```python
from build123d import *

# Parameters (mm, degrees)
SALIENTE_EXTRUIR1_DEPTH = 14
CROQUIS7_W              = 84
CROQUIS7_H              = 14.5
SALIENTE_EXTRUIR6_DEPTH = 3
SALIENTE_EXTRUIR7_DEPTH = 5
REDONDEO1_R             = 2


with BuildPart() as part:
    # Croquis1 → Saliente-Extruir1 (new body)
    with BuildSketch(Plane.XY):
        Polygon((-38.5, 7.25), (-42, 7.25), (-42, -7.25), (42, -7.25), (42, 7.25), (38.5, 7.25), (38.5, -2.25), (-38.5, -2.25), align=None)
    extrude(amount=SALIENTE_EXTRUIR1_DEPTH)

    # Croquis7 → Saliente-Extruir6 (add)
    with BuildSketch(Plane.XY.offset(14)):
        Rectangle(CROQUIS7_W, CROQUIS7_H)
    extrude(amount=SALIENTE_EXTRUIR6_DEPTH)

    # Croquis8 → Saliente-Extruir7 (add)
    with BuildSketch(Plane(origin=(0, 0, 0), x_dir=(-1, 0, 0), z_dir=(0, 0, -1))):
        Polygon((-42, 7.25), (-42, -7.25), (42, -7.25), (42, 7.25), (38.5, 7.25), (38.5, -2.25), (-38.5, -2.25), (-38.5, 7.25), align=None)
    extrude(amount=SALIENTE_EXTRUIR7_DEPTH)

    # Redondeo1
    redondeo1_edges = [part.edges().sort_by_distance(p)[0] for p in [
        (-38.5, -2.25, 4.5),
        (38.5, -2.25, 4.5),
        (-42, 0, 17),
        (42, 0, 17),
        (42, 0, -5),
        (-42, 0, -5),
    ]]
    fillet(redondeo1_edges, radius=REDONDEO1_R)


solid = part.part
```
Geometry: final body of the model. Coordinates: model frame, mm. A direction names the side the tool comes from. Round coordinates to 2 decimals unless told otherwise and drop trailing zeros. Order: outer loops, then holes, each group sorted by start corner. A loop starts at its lowest first (then second) coordinate and runs counter-clockwise, first axis right, second up. Notation, with made-up numbers: (34, -8.75) - (71, -8.75) arc R26 ccw to (71, 20.25) - close; hole circle Ø5 at (-36, 81). An arc over 180 degrees is marked (long way). Write item = value, one per line. Start each with the question number.
Q1. Pull-direction query (X, two-part tool) for faces 3 (the cylindrical face through (-37.9, -1.68, 4.37)), 4 (the flat face through (42, 0, 6)), 5 (the cylindrical face through (-41.4, 0.1, 16.43)); classes: +X half, -X half, draft (parallel to the pull), parting line (faces both ways), or undercut.
Q2. Cut plane A-A on z = 1. Return the cut outline in (x, y), and give its area (3 significant figures).
Q3. Pin query (flat end, axial travel): pin 1 (9.5 mm diameter, centred on x = -13, z = 9, fed in from +Y); pin 2 (3 mm diameter, centred on x = -16, y = 2, fed in from -Z). Return the tip coordinate at first contact, or that it passes through.
Q4. Cut plane C-C on x = -3. Return the cut outline in (y, z), and give its area (4 significant figures).
Q5. Ray query, line 1 (X direction, y = 6.25, z = 7); line 2 (Z direction, x = 19.5, y = -1.5); line 3 (X direction, y = -2, z = 0.75). Return the intervals inside material, ascending. Write a range as from..to.
Q6. Access query for faces 1 (the flat face through (38.5, 3, 5)), 2 (the cylindrical face through (41.43, 0.1, 16.4)). Directions: +Z, -Z, +X, -X, +Y, -Y. A direction counts if a zero-diameter tool reaches every point of the face in a straight line with its end or side. Return the directions, or none.
Q7. Cut plane B-B on y = 6. Return the cut outline in (x, z).
Outcome:
q1.face_3 = undercut
q1.face_4 = +X half
q1.face_5 = -X half
q2.outline = (-42, -7.25) - (42, -7.25) - (42, 7.25) - (38.5, 7.25) - (38.5, -0.25) arc R2 cw to (36.5, -2.25) - (-36.5, -2.25) arc R2 cw to (-38.5, -0.25) - (-38.5, 7.25) - (-42, 7.25) - close
q2.area = 488 mm^2
q3.pin_1 = -2.25
q3.pin_2 = 14
q4.outline = (-7.25, -5) - (-2.25, -5) - (-2.25, 14) - (7.25, 14) - (7.25, 17) - (-7.25, 17) - close
q4.area = 138.5 mm^2
q5.line_1 = -42..-38.5, 38.5..42
q5.line_2 = 14..17
q5.line_3 = -42..-37.47, 37.47..42
q6.face_1 = -Z, +Y
q6.face_2 = +Z, +X, +Y, -Y
q7.outline = (-42, -3) arc R2 ccw to (-40, -5) - (-38.5, -5) - (-38.5, 14) - (38.5, 14) - (38.5, -5) - (40, -5) arc R2 ccw to (42, -3) - (42, 15) arc R2 ccw to (40, 17) - (-40, 17) arc R2 ccw to (-42, 15) - close
